from build123d import *

# Parameters (mm, degrees)
BOSS_EXTRUDE1_DEPTH = 30


with BuildPart() as part:
    # Sketch1 → Boss-Extrude1 (new body)
    with BuildSketch(Plane.XY):
        with BuildLine():
            Line((-3.487823687, 49.878202513), (-10.463471062, 149.634607539))
            ThreePointArc((-10.463471062, 149.634607539), (0, 150), (10.463471062, 149.634607539))
            Line((10.463471062, 149.634607539), (3.487823687, 49.878202513))
            ThreePointArc((3.487823687, 49.878202513), (4.900857016, 49.759236334), (6.309948457, 49.600247484))
            Line((6.309948457, 49.600247484), (18.92984537, 148.800742452))
            ThreePointArc((18.92984537, 148.800742452), (29.263548302, 147.11779206), (39.454682169, 144.718098574))
            Line((39.454682169, 144.718098574), (13.151560723, 48.239366191))
            ThreePointArc((13.151560723, 48.239366191), (14.514233863, 47.847016787), (15.86523282, 47.41618276))
            Line((15.86523282, 47.41618276), (47.595698461, 142.248548281))
            ThreePointArc((47.595698461, 142.248548281), (57.402514855, 138.581929877), (66.929671966, 134.24015424))
            Line((66.929671966, 134.24015424), (22.309890655, 44.74671808))
            ThreePointArc((22.309890655, 44.74671808), (23.569836841, 44.096063217), (24.810825184, 43.409940724))
            Line((24.810825184, 43.409940724), (74.432475551, 130.229822173))
            ThreePointArc((74.432475551, 130.229822173), (83.335534953, 124.720441845), (91.832592005, 118.603436062))
            Line((91.832592005, 118.603436062), (30.610864002, 39.534478687))
            ThreePointArc((30.610864002, 39.534478687), (31.719664208, 38.650522668), (32.80295145, 37.735479011))
            Line((32.80295145, 37.735479011), (98.408854349, 113.206437033))
            ThreePointArc((98.408854349, 113.206437033), (106.066017178, 106.066017178), (113.206437033, 98.408854349))
            Line((113.206437033, 98.408854349), (37.735479011, 32.80295145))
            ThreePointArc((37.735479011, 32.80295145), (38.650522668, 31.719664208), (39.534478687, 30.610864002))
            Line((39.534478687, 30.610864002), (118.603436062, 91.832592005))
            ThreePointArc((118.603436062, 91.832592005), (124.720441845, 83.335534953), (130.229822173, 74.432475551))
            Line((130.229822173, 74.432475551), (43.409940724, 24.810825184))
            ThreePointArc((43.409940724, 24.810825184), (44.096063217, 23.569836841), (44.74671808, 22.309890655))
            Line((44.74671808, 22.309890655), (134.24015424, 66.929671966))
            ThreePointArc((134.24015424, 66.929671966), (138.581929877, 57.402514855), (142.248548281, 47.595698461))
            Line((142.248548281, 47.595698461), (47.41618276, 15.86523282))
            ThreePointArc((47.41618276, 15.86523282), (47.847016787, 14.514233863), (48.239366191, 13.151560723))
            Line((48.239366191, 13.151560723), (144.718098574, 39.454682169))
            ThreePointArc((144.718098574, 39.454682169), (147.11779206, 29.263548302), (148.800742452, 18.92984537))
            Line((148.800742452, 18.92984537), (49.600247484, 6.309948457))
            ThreePointArc((49.600247484, 6.309948457), (49.759236334, 4.900857016), (49.878202513, 3.487823687))
            Line((49.878202513, 3.487823687), (149.634607539, 10.463471062))
            ThreePointArc((149.634607539, 10.463471062), (150, 0), (149.634607539, -10.463471062))
            Line((149.634607539, -10.463471062), (49.878202513, -3.487823687))
            ThreePointArc((49.878202513, -3.487823687), (49.759236334, -4.900857016), (49.600247484, -6.309948457))
            Line((49.600247484, -6.309948457), (148.800742452, -18.92984537))
            ThreePointArc((148.800742452, -18.92984537), (147.11779206, -29.263548302), (144.718098574, -39.454682169))
            Line((144.718098574, -39.454682169), (48.239366191, -13.151560723))
            ThreePointArc((48.239366191, -13.151560723), (47.847016787, -14.514233863), (47.41618276, -15.86523282))
            Line((47.41618276, -15.86523282), (142.248548281, -47.595698461))
            ThreePointArc((142.248548281, -47.595698461), (138.581929877, -57.402514855), (134.24015424, -66.929671966))
            Line((134.24015424, -66.929671966), (44.74671808, -22.309890655))
            ThreePointArc((44.74671808, -22.309890655), (44.096063217, -23.569836841), (43.409940724, -24.810825184))
            Line((43.409940724, -24.810825184), (130.229822173, -74.432475551))
            ThreePointArc((130.229822173, -74.432475551), (124.720441845, -83.335534953), (118.603436062, -91.832592005))
            Line((118.603436062, -91.832592005), (39.534478687, -30.610864002))
            ThreePointArc((39.534478687, -30.610864002), (38.650522668, -31.719664208), (37.735479011, -32.80295145))
            Line((37.735479011, -32.80295145), (113.206437033, -98.408854349))
            ThreePointArc((113.206437033, -98.408854349), (106.066017178, -106.066017178), (98.408854349, -113.206437033))
            Line((98.408854349, -113.206437033), (32.80295145, -37.735479011))
            ThreePointArc((32.80295145, -37.735479011), (31.719664208, -38.650522668), (30.610864002, -39.534478687))
            Line((30.610864002, -39.534478687), (91.832592005, -118.603436062))
            ThreePointArc((91.832592005, -118.603436062), (83.335534953, -124.720441845), (74.432475551, -130.229822173))
            Line((74.432475551, -130.229822173), (24.810825184, -43.409940724))
            ThreePointArc((24.810825184, -43.409940724), (23.569836841, -44.096063217), (22.309890655, -44.74671808))
            Line((22.309890655, -44.74671808), (66.929671966, -134.24015424))
            ThreePointArc((66.929671966, -134.24015424), (57.402514855, -138.581929877), (47.595698461, -142.248548281))
            Line((47.595698461, -142.248548281), (15.86523282, -47.41618276))
            ThreePointArc((15.86523282, -47.41618276), (14.514233863, -47.847016787), (13.151560723, -48.239366191))
            Line((13.151560723, -48.239366191), (39.454682169, -144.718098574))
            ThreePointArc((39.454682169, -144.718098574), (29.263548302, -147.11779206), (18.92984537, -148.800742452))
            Line((18.92984537, -148.800742452), (6.309948457, -49.600247484))
            ThreePointArc((6.309948457, -49.600247484), (4.900857016, -49.759236334), (3.487823687, -49.878202513))
            Line((3.487823687, -49.878202513), (10.463471062, -149.634607539))
            ThreePointArc((10.463471062, -149.634607539), (0, -150), (-10.463471062, -149.634607539))
            Line((-10.463471062, -149.634607539), (-3.487823687, -49.878202513))
            ThreePointArc((-3.487823687, -49.878202513), (-4.900857016, -49.759236334), (-6.309948457, -49.600247484))
            Line((-6.309948457, -49.600247484), (-18.92984537, -148.800742452))
            ThreePointArc((-18.92984537, -148.800742452), (-29.263548302, -147.11779206), (-39.454682169, -144.718098574))
            Line((-39.454682169, -144.718098574), (-13.151560723, -48.239366191))
            ThreePointArc((-13.151560723, -48.239366191), (-14.514233863, -47.847016787), (-15.86523282, -47.41618276))
            Line((-15.86523282, -47.41618276), (-47.595698461, -142.248548281))
            ThreePointArc((-47.595698461, -142.248548281), (-57.402514855, -138.581929877), (-66.929671966, -134.24015424))
            Line((-66.929671966, -134.24015424), (-22.309890655, -44.74671808))
            ThreePointArc((-22.309890655, -44.74671808), (-23.569836841, -44.096063217), (-24.810825184, -43.409940724))
            Line((-24.810825184, -43.409940724), (-74.432475551, -130.229822173))
            ThreePointArc((-74.432475551, -130.229822173), (-83.335534953, -124.720441845), (-91.832592005, -118.603436062))
            Line((-91.832592005, -118.603436062), (-30.610864002, -39.534478687))
            ThreePointArc((-30.610864002, -39.534478687), (-31.719664208, -38.650522668), (-32.80295145, -37.735479011))
            Line((-32.80295145, -37.735479011), (-98.408854349, -113.206437033))
            ThreePointArc((-98.408854349, -113.206437033), (-106.066017178, -106.066017178), (-113.206437033, -98.408854349))
            Line((-113.206437033, -98.408854349), (-37.735479011, -32.80295145))
            ThreePointArc((-37.735479011, -32.80295145), (-38.650522668, -31.719664208), (-39.534478687, -30.610864002))
            Line((-39.534478687, -30.610864002), (-118.603436062, -91.832592005))
            ThreePointArc((-118.603436062, -91.832592005), (-124.720441845, -83.335534953), (-130.229822173, -74.432475551))
            Line((-130.229822173, -74.432475551), (-43.409940724, -24.810825184))
            ThreePointArc((-43.409940724, -24.810825184), (-44.096063217, -23.569836841), (-44.74671808, -22.309890655))
            Line((-44.74671808, -22.309890655), (-134.24015424, -66.929671966))
            ThreePointArc((-134.24015424, -66.929671966), (-138.581929877, -57.402514855), (-142.248548281, -47.595698461))
            Line((-142.248548281, -47.595698461), (-47.41618276, -15.86523282))
            ThreePointArc((-47.41618276, -15.86523282), (-47.847016787, -14.514233863), (-48.239366191, -13.151560723))
            Line((-48.239366191, -13.151560723), (-144.718098574, -39.454682169))
            ThreePointArc((-144.718098574, -39.454682169), (-147.11779206, -29.263548302), (-148.800742452, -18.92984537))
            Line((-148.800742452, -18.92984537), (-49.600247484, -6.309948457))
            ThreePointArc((-49.600247484, -6.309948457), (-49.759236334, -4.900857016), (-49.878202513, -3.487823687))
            Line((-49.878202513, -3.487823687), (-149.634607539, -10.463471062))
            ThreePointArc((-149.634607539, -10.463471062), (-150, 0), (-149.634607539, 10.463471062))
            Line((-149.634607539, 10.463471062), (-49.878202513, 3.487823687))
            ThreePointArc((-49.878202513, 3.487823687), (-49.759236334, 4.900857016), (-49.600247484, 6.309948457))
            Line((-49.600247484, 6.309948457), (-148.800742452, 18.92984537))
            ThreePointArc((-148.800742452, 18.92984537), (-147.11779206, 29.263548302), (-144.718098574, 39.454682169))
            Line((-144.718098574, 39.454682169), (-48.239366191, 13.151560723))
            ThreePointArc((-48.239366191, 13.151560723), (-47.847016787, 14.514233863), (-47.41618276, 15.86523282))
            Line((-47.41618276, 15.86523282), (-142.248548281, 47.595698461))
            ThreePointArc((-142.248548281, 47.595698461), (-138.581929877, 57.402514855), (-134.24015424, 66.929671966))
            Line((-134.24015424, 66.929671966), (-44.74671808, 22.309890655))
            ThreePointArc((-44.74671808, 22.309890655), (-44.096063217, 23.569836841), (-43.409940724, 24.810825184))
            Line((-43.409940724, 24.810825184), (-130.229822173, 74.432475551))
            ThreePointArc((-130.229822173, 74.432475551), (-124.720441845, 83.335534953), (-118.603436062, 91.832592005))
            Line((-118.603436062, 91.832592005), (-39.534478687, 30.610864002))
            ThreePointArc((-39.534478687, 30.610864002), (-38.650522668, 31.719664208), (-37.735479011, 32.80295145))
            Line((-37.735479011, 32.80295145), (-113.206437033, 98.408854349))
            ThreePointArc((-113.206437033, 98.408854349), (-106.066017178, 106.066017178), (-98.408854349, 113.206437033))
            Line((-98.408854349, 113.206437033), (-32.80295145, 37.735479011))
            ThreePointArc((-32.80295145, 37.735479011), (-31.719664208, 38.650522668), (-30.610864002, 39.534478687))
            Line((-30.610864002, 39.534478687), (-91.832592005, 118.603436062))
            ThreePointArc((-91.832592005, 118.603436062), (-83.335534953, 124.720441845), (-74.432475551, 130.229822173))
            Line((-74.432475551, 130.229822173), (-24.810825184, 43.409940724))
            ThreePointArc((-24.810825184, 43.409940724), (-23.569836841, 44.096063217), (-22.309890655, 44.74671808))
            Line((-22.309890655, 44.74671808), (-66.929671966, 134.24015424))
            ThreePointArc((-66.929671966, 134.24015424), (-57.402514855, 138.581929877), (-47.595698461, 142.248548281))
            Line((-47.595698461, 142.248548281), (-15.86523282, 47.41618276))
            ThreePointArc((-15.86523282, 47.41618276), (-14.514233863, 47.847016787), (-13.151560723, 48.239366191))
            Line((-13.151560723, 48.239366191), (-39.454682169, 144.718098574))
            ThreePointArc((-39.454682169, 144.718098574), (-29.263548302, 147.11779206), (-18.92984537, 148.800742452))
            Line((-18.92984537, 148.800742452), (-6.309948457, 49.600247484))
            ThreePointArc((-6.309948457, 49.600247484), (-4.900857016, 49.759236334), (-3.487823687, 49.878202513))
        make_face()
    extrude(amount=BOSS_EXTRUDE1_DEPTH)


solid = part.part
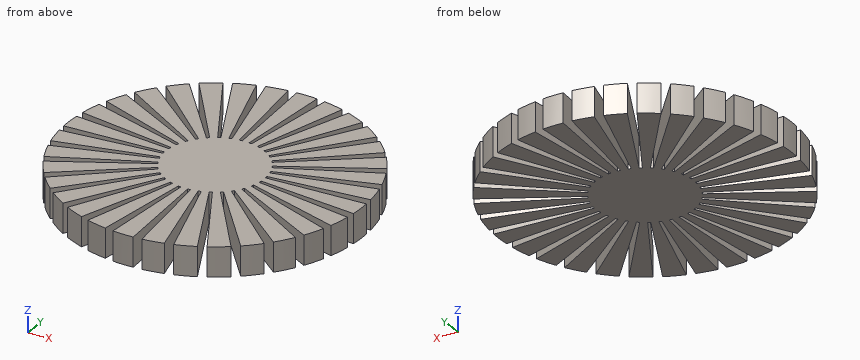
Geometry: final body of the model. Coordinates: model frame, mm. Give positions to 0.01 mm unless a question says otherwise; leave off trailing zeros. Write each loop counter-clockwise with the first axis right and the second up, starting at its lowest first coordinate (ties: lowest second). Pieces come first, ordered by that corner, then holes. Notation, with made-up numbers: M 15,-1.75 L 32,-1.75 A11 ccw 32,6.25 Z; hole C 48.25,77.25 d5. An arc over 180 degrees is marked long. Answer in a Markdown table with one row per item. Add a question column.
(1) First-contact query: pin 1 (1 mm diameter, centred on y = -108, z = 27, fed in from +X); pin 2 (8 mm diameter, centred on x = -79.5, z = 25, fed in from -Y); pin 3 (4 mm diameter, centred on y = -63, z = 16, fed in from -X); pin 4 (5 mm diameter, centred on x = -119, y = -94, fed in from -Z). Flat tips, straight axial feed; report the tip coordinate or a pass-through.
(2) Section B-B on x = 79. State how many separate pieces and enclosed holes the cut face has, and give its area (3 significant figures).
(3) Ray query, line 1 (Y direction, x = -131.5, z = 4.5); line 2 (X direction, y = 135, z = 12.5). Return the intervals inside material, ascending.
(4) Section A-A on y = 124.5. Return loops of the section in (x, z), and give its area (3 significant figures).
Result set:
| question | item | result |
|---|---|---|
| 1 | pin 1 | stops at x = 104.61 |
| 1 | pin 2 | stops at y = -129.61 |
| 1 | pin 3 | stops at x = -137.04 |
| 1 | pin 4 | stops at z = 0 |
| 2 | separate pieces | 11 |
| 2 | enclosed holes | 0 |
| 2 | area | 5,620 mm^2 |
| 3 | line 1 | y = -65.56 to -44, -35.85 to -16.73, -9.2 to 9.2, 16.73 to 35.85, 44 to 65.56 |
| 3 | line 2 | x = -65.38 to -45.17, -36.81 to -17.17, -9.44 to 9.44, 17.17 to 36.81, 45.17 to 65.38 |
| 4 | outline | M -83.66,0 L -71.16,0 L -71.16,30 L -83.66,30 Z; M -62.07,0 L -41.66,0 L -41.66,30 L -62.07,30 Z; M -33.94,0 L -15.84,0 L -15.84,30 L -33.94,30 Z; M -8.71,0 L 8.71,0 L 8.71,30 L -8.71,30 Z; M 15.84,0 L 33.94,0 L 33.94,30 L 15.84,30 Z; M 41.66,0 L 62.07,0 L 62.07,30 L 41.66,30 Z; M 71.16,0 L 83.66,0 L 83.66,30 L 71.16,30 Z |
| 4 | area | 3,580 mm^2 |
